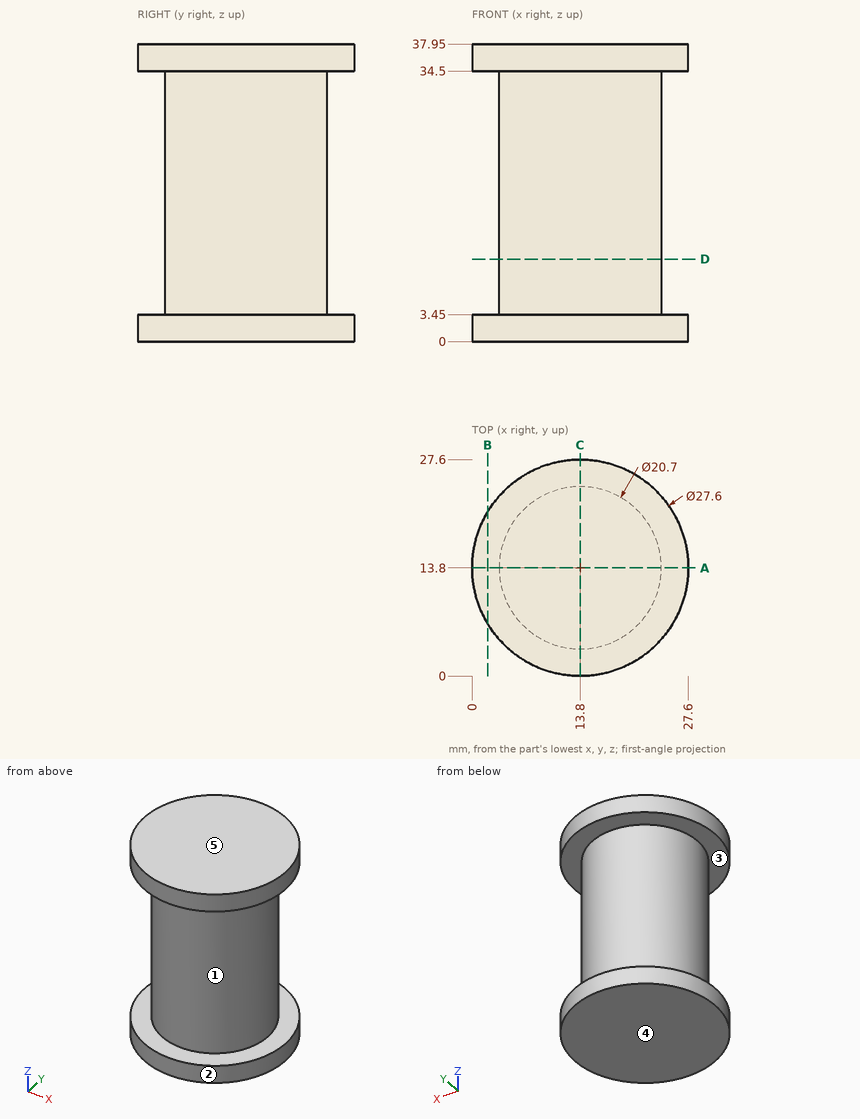
Study the drawing (mm; zero at the part's minimum x, y, z) and answer. A direction names the side the tool comes from. Coordinates: 2 decimals unless noted, no trailing zeros. Write each loop counter-clockwise with the first axis right and the second up, starting at its lowest first coordinate (ties: lowest second). Pieces come first, ordered by that corner, then holes. Notation, with made-up numbers: M -4.75,28.5 L 20.25,28.5 A26 cw 20.25,58.5 Z; hole C -6,63 d8. An arc over 180 degrees is marked long. Write each question's results on one line, items separated by ' | '.
Item 1: The part is cut by section A-A on y = 13.8. Determine the outline of the cut face in (x, z), and give its area (3 significant figures).
Answer below:
outline: M 0,0 L 27.6,0 L 27.6,3.45 L 24.15,3.45 L 24.15,34.5 L 27.6,34.5 L 27.6,37.95 L 0,37.95 L 0,34.5 L 3.45,34.5 L 3.45,3.45 L 0,3.45 Z | area: 833 mm2
Item 2: Given P1, Ø4, axis at y = 12, z = 28.5, coming from the -X side; P2, Ø5, axis at x = 20.5, z = 30, coming from the -Y side; P3, Ø2, axis at y = 10, z = 15, coming from the -X side; P4, Ø12, axis at x = 17, y = 24.5, coming from the -Z side, each flat-ended and moving along its own axis, determine where each tip first touches the part or whether it passes through.
Answer below:
P1: x = 3.45 | P2: y = 4.34 | P3: x = 3.84 | P4: z = 0
Item 3: Consider probe 1 along Z at (x, y) = (26.25, 12.75); probe 2 along Y at (x, z) = (19.25, 24); probe 3 along Y at (x, z) = (8.25, 31.5). Determine where each line is inside the solid, lowest interval first. Write a range as [from, to].
Answer below:
probe 1: [0, 3.45], [34.5, 37.95] | probe 2: [5, 22.6] | probe 3: [5.06, 22.54]
Item 4: The part is cut by section D-D on z = 10.5. Determine the outline of the cut face in (x, y), and give its area (3 significant figures).
Answer below:
outline: C 13.8,13.8 d20.7 | area: 337 mm2
Item 5: For a pull along Z with two mould halves and no side action, classify the marked faces 3, 4 and 5 as released by +Z, released by -Z, zero draft, split by the parting line, or undercut.
Answer below:
face 3: undercut | face 4: released by -Z | face 5: released by +Z
Item 6: The part is cut by section B-B on x = 2. Determine the outline of the cut face in (y, z), and give its area (3 significant figures).
Answer below:
outline: M 6.64,0 L 20.96,0 L 20.96,3.45 L 6.64,3.45 Z; M 6.64,34.5 L 20.96,34.5 L 20.96,37.95 L 6.64,37.95 Z | area: 98.7 mm2
Item 7: Which of the six approach directions +Z, -Z, +X, -X, +Y, -Y give full straight-line access (tool end or side, diameter ignored) to the marked faces 1 and 2?
Answer below:
face 1: none | face 2: +Z, -Z
